Geometry check sheet. Reference: the model listing, model coordinates, mm. Give positions to 0.01 mm unless a question says otherwise; leave off trailing zeros. Write each loop counter-clockwise with the first axis right and the second up, starting at its lowest first coordinate (ties: lowest second). Pieces come first, ordered by that corner, then holes. Notation, with made-up numbers: (61.25, 75.25) - (94.25, 75.25) arc R11 cw to (94.25, 81.25) - close; hole circle Ø11 at (52.25, -27). An arc over 180 degrees is marked (long way). Write item = value, one per line. Start each with the question number.
(1) Section check C-C, the plane z = -3.1. Enter the section's corners in (x, y) (3 decimals), plus the area to 3 significant figures.
(2) Section check D-D, the plane x = -46. Enter the section's corners in (y, z), plus the area to 3 significant figures.
(3) Depth check by flat-ended pin: pin 1 Ø1 at (x, z) = (93.5, -2) entering from +Y; pin 2 Ø2 at (x, z) = (83.5, -1.5) entering from +Y; pin 3 Ø4 at (x, y) = (103, -59) entering from +Z; pin 4 Ø2 at (y, z) = (-76.5, -1) entering from +X. Enter the tip coordinate at first touch or a pass-through.
(4) Thickness scan on L1, parallel to Y at x = -41, z = -1.3; L2, parallel to Y at x = -40.5, z = -1.65; L3, parallel to X at y = -74.5, z = -2.85. Record the ranges inside material, lowest first.
(5) Section check B-B, the plane y = 0. Enter the section's corners in (x, z) (3 decimals), plus the area to 3 significant figures.
(6) Section check A-A, the plane x = 0. Enter the section's corners in (y, z) (3 decimals), plus the area to 3 significant figures.
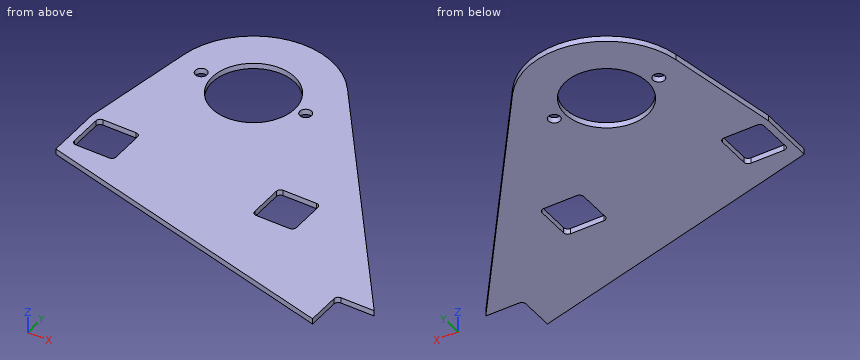
```python
from build123d import *

# Parameters (mm, degrees)
SKETCH_1_R             = 4.25
SKETCH_1_R_2           = 29.732137495
SM_BASE_FLANGE_1_DEPTH = 4


# Sheet-metal steps are written as plain solids
with BuildPart() as part:
    # Sketch 1 → Базовая кромка1 (new body)
    with BuildSketch(Plane.XY):
        with BuildLine():
            Line((179.733197448, -143.22618932), (45.492707493, 34.38406884))
            ThreePointArc((45.492707493, 34.38406884), (-13.549825845, 55.391812072), (-56.227876086, 9.501398625))
            Line((-56.227876086, 9.501398625), (-70, -72))
            Line((-70, -72), (-70, -112))
            Line((-70, -112), (152.733197448, -170.22618932))
            Line((152.733197448, -170.22618932), (152.733197448, -146.22618932))
            ThreePointArc((152.733197448, -146.22618932), (153.611877105, -144.104868976), (155.733197448, -143.22618932))
            Line((155.733197448, -143.22618932), (179.733197448, -143.22618932))
        make_face()
        with Locations((-37.675, 0)):
            Circle(SKETCH_1_R, mode=Mode.SUBTRACT)
        Circle(SKETCH_1_R_2, mode=Mode.SUBTRACT)
        with Locations((37.675, 0)):
            Circle(SKETCH_1_R, mode=Mode.SUBTRACT)
        with BuildLine():
            Line((-62, -102), (-38, -102))
            ThreePointArc((-38, -102), (-35.878679656, -101.121320344), (-35, -99))
            Line((-35, -99), (-35, -75))
            ThreePointArc((-35, -75), (-35.878679656, -72.878679656), (-38, -72))
            Line((-38, -72), (-62, -72))
            ThreePointArc((-62, -72), (-64.121320344, -72.878679656), (-65, -75))
            Line((-65, -75), (-65, -99))
            ThreePointArc((-65, -99), (-64.121320344, -101.121320344), (-62, -102))
        make_face(mode=Mode.SUBTRACT)
        with BuildLine():
            Line((68, -102), (92, -102))
            ThreePointArc((92, -102), (94.121320344, -101.121320344), (95, -99))
            Line((95, -99), (95, -75))
            ThreePointArc((95, -75), (94.121320344, -72.878679656), (92, -72))
            Line((92, -72), (68, -72))
            ThreePointArc((68, -72), (65.878679656, -72.878679656), (65, -75))
            Line((65, -75), (65, -99))
            ThreePointArc((65, -99), (65.878679656, -101.121320344), (68, -102))
        make_face(mode=Mode.SUBTRACT)
    extrude(amount=-SM_BASE_FLANGE_1_DEPTH)


solid = part.part
```
Model answer:
q1.outline = (-70, -112) - (152.733, -170.226) - (152.733, -146.226) arc R3 cw to (155.733, -143.226) - (179.733, -143.226) - (45.493, 34.384) arc R57.025 ccw to (-56.228, 9.501) - (-70, -72) - close; hole (-65, -99) arc R3 ccw to (-62, -102) - (-38, -102) arc R3 ccw to (-35, -99) - (-35, -75) arc R3 ccw to (-38, -72) - (-62, -72) arc R3 ccw to (-65, -75) - close; hole circle Ø8.5 at (-37.675, 0); hole circle Ø59.464 at (0, 0); hole circle Ø8.5 at (37.675, 0); hole (65, -99) arc R3 ccw to (68, -102) - (92, -102) arc R3 ccw to (95, -99) - (95, -75) arc R3 ccw to (92, -72) - (68, -72) arc R3 ccw to (65, -75) - close
q1.area = 27,700 mm²
q2.outline = (-118.27, -4) - (-102, -4) - (-102, 0) - (-118.27, 0) - close; (-72, -4) - (33.7, -4) - (33.7, 0) - (-72, 0) - close
q2.area = 488 mm²
q3.pin_1 = -28.47
q3.pin_2 = -14.58
q3.pin_3 = 0
q3.pin_4 = 130.06
q4.L1 = -119.58 to -102, -72 to -2.65, 2.65 to 39.63
q4.L2 = -119.71 to -102, -72 to -3.18, 3.18 to 40.14
q4.L3 = -70 to -64.96, -35.04 to 65.04, 94.96 to 127.79
q5.outline = (-57.833, -4) - (-41.925, -4) - (-41.925, 0) - (-57.833, 0) - close; (-33.425, -4) - (-29.732, -4) - (-29.732, 0) - (-33.425, 0) - close; (29.732, -4) - (33.425, -4) - (33.425, 0) - (29.732, 0) - close; (41.925, -4) - (71.481, -4) - (71.481, 0) - (41.925, 0) - close
q5.area = 211 mm²
q6.outline = (-130.299, -4) - (-29.732, -4) - (-29.732, 0) - (-130.299, 0) - close; (29.732, -4) - (57.025, -4) - (57.025, 0) - (29.732, 0) - close
q6.area = 511 mm²
